Check sheet for the modelled part. Datum: model origin and axes. Units: mm. Round coordinates to 2 decimals unless told otherwise and drop trailing zeros. Order: outer loops, then holes, each group sorted by start corner. A loop starts at its lowest first (then second) coordinate and runs counter-clockwise, first axis right, second up. Notation, with made-up numbers: M -34.75,-11 L -2.75,-11 A20 cw -2.75,-4 Z; hole C -33.5,33 d8. An arc over 180 degrees is marked long. One line per item, written item: value. Start each with the question number.
(1) Depth check by flat-ended pin: pin 1 Ø1 at (y, z) = (-13.5, -3.5) entering from +X; pin 2 Ø12 at (x, z) = (11, -7.5) entering from +Y; pin 3 Ø2 at (x, y) = (9, -13) entering from -Z; pin 4 Ø2 at (x, y) = (-3, -4) entering from -Z. Enter the tip coordinate at first touch or a pass-through.
(2) Cross-section at B-B, the plane z = 31. Enter the section's corners in (x, y).
(3) Cross-section at D-D, the plane x = -2.25. Enter the section's corners in (y, z), and give its area (3 significant figures).
(4) Cross-section at C-C, the plane x = 3.5. Enter the section's corners in (y, z).
(5) Thickness scan on L1, parallel to X at y = -6.5, z = 38.1; L2, parallel to Z at x = 3, y = -13.5; L3, parallel to Z at x = 9.5, y = -3.5. Record the ranges inside material, lowest first.
(6) Cross-section at A-A, the plane y = -9.25. Enter the section's corners in (x, z).
from build123d import *

# Parameters (mm, degrees)
F1_DEPTH = 15.24


with BuildPart() as f1:
    # F0 (on Front) → F1 (new body)
    with BuildSketch(Plane.XZ):
        with BuildLine():
            ThreePointArc((-10.9982, 0), (-7.776902, 7.776902), (0, 10.9982))
            Line((0, 10.9982), (0, 24.13))
            ThreePointArc((0, 24.13), (-9.485208, 27.843698), (-13.927438, 37.01034))
            Line((-13.927438, 37.01034), (-13.97, 0))
            Line((-13.97, 0), (-10.9982, 0))
        make_face()
        with BuildLine():
            Line((0, 24.13), (0, 10.9982))
            ThreePointArc((0, 10.9982), (7.776902, 7.776902), (10.9982, 0))
            Line((10.9982, 0), (13.97, 0))
            Line((13.97, 0), (13.927438, 37.01034))
            ThreePointArc((13.927438, 37.01034), (9.485208, 27.843698), (0, 24.13))
        make_face()
        with BuildLine():
            Line((0, -24.13), (0, -10.9982))
            ThreePointArc((0, -10.9982), (-7.776902, -7.776902), (-10.9982, 0))
            Line((-10.9982, 0), (-13.97, 0))
            Line((-13.97, 0), (-13.927438, -37.01034))
            ThreePointArc((-13.927438, -37.01034), (-9.485208, -27.843698), (0, -24.13))
        make_face()
        with BuildLine():
            ThreePointArc((10.9982, 0), (7.776902, -7.776902), (0, -10.9982))
            Line((0, -10.9982), (0, -24.13))
            ThreePointArc((0, -24.13), (9.485208, -27.843698), (13.927438, -37.01034))
            Line((13.927438, -37.01034), (13.97, 0))
            Line((13.97, 0), (10.9982, 0))
        make_face()
        with BuildLine():
            ThreePointArc((10.9982, 38.1), (-7.776902, 45.876902), (0, 27.1018))
            ThreePointArc((0, 27.1018), (7.776902, 30.323098), (10.9982, 38.1))
        make_face()
        with BuildLine():
            ThreePointArc((-13.927438, 37.01034), (-9.485208, 27.843698), (0, 24.13))
            ThreePointArc((0, 24.13), (9.485208, 27.843698), (13.927438, 37.01034))
            ThreePointArc((13.927438, 37.01034), (13.959356, 37.554755), (13.97, 38.1))
            ThreePointArc((13.97, 38.1), (-0.545245, 52.059356), (-13.927438, 37.01034))
        make_face()
        with BuildLine():
            ThreePointArc((10.9982, 38.1), (7.776902, 30.323098), (0, 27.1018))
            ThreePointArc((0, 27.1018), (-7.776902, 45.876902), (10.9982, 38.1))
        make_face(mode=Mode.SUBTRACT)
        with BuildLine():
            ThreePointArc((10.9982, -38.1), (7.776902, -30.323098), (0, -27.1018))
            ThreePointArc((0, -27.1018), (-7.776902, -45.876902), (10.9982, -38.1))
        make_face()
        with BuildLine():
            ThreePointArc((13.927438, -37.01034), (9.485208, -27.843698), (0, -24.13))
            ThreePointArc((0, -24.13), (-9.485208, -27.843698), (-13.927438, -37.01034))
            ThreePointArc((-13.927438, -37.01034), (-0.545245, -52.059356), (13.97, -38.1))
            ThreePointArc((13.97, -38.1), (13.959356, -37.554755), (13.927438, -37.01034))
        make_face()
        with BuildLine():
            ThreePointArc((10.9982, -38.1), (-7.776902, -45.876902), (0, -27.1018))
            ThreePointArc((0, -27.1018), (7.776902, -30.323098), (10.9982, -38.1))
        make_face(mode=Mode.SUBTRACT)
    extrude(amount=F1_DEPTH)


solid = f1.part
Values found:
1. pin 1: x = 13.97
1. pin 2: y = 0
1. pin 3: z = -49.55
1. pin 4: z = -51.93
2. outline: M -13.93,-15.24 L -8.4,-15.24 L -8.4,0 L -13.93,0 Z; M 8.4,-15.24 L 13.93,-15.24 L 13.93,0 L 8.4,0 Z
3. outline: M -15.24,-51.89 L 0,-51.89 L 0,-48.87 L -15.24,-48.87 Z; M -15.24,-27.33 L 0,-27.33 L 0,-10.77 L -15.24,-10.77 Z; M -15.24,10.77 L 0,10.77 L 0,27.33 L -15.24,27.33 Z; M -15.24,48.87 L 0,48.87 L 0,51.89 L -15.24,51.89 Z
3. area: 597 mm^2
4. outline: M -15.24,-51.62 L 0,-51.62 L 0,-48.53 L -15.24,-48.53 Z; M -15.24,-27.67 L 0,-27.67 L 0,-10.43 L -15.24,-10.43 Z; M -15.24,10.43 L 0,10.43 L 0,27.67 L -15.24,27.67 Z; M -15.24,48.53 L 0,48.53 L 0,51.62 L -15.24,51.62 Z
5. L1: -13.97 to -11, 11 to 13.97
5. L2: -51.74 to -48.68, -27.52 to -10.58, 10.58 to 27.52, 48.68 to 51.74
5. L3: -48.34 to -43.64, -32.56 to -5.54, 5.54 to 32.56, 43.64 to 48.34
6. outline: M -13.97,0 L -13.93,-37.01 A13.97 ccw long 13.97,-38.1 A13.97 ccw 13.93,-37.01 L 13.97,0 L 13.93,37.01 A13.97 ccw 13.97,38.1 A13.97 ccw long -13.93,37.01 Z; hole C 0,-38.1 d22; hole M -11,0 A11 ccw 0,-11 A11 ccw 11,0 A11 ccw 0,11 A11 ccw Z; hole C 0,38.1 d22
